from build123d import *

# Parameters (mm, degrees)
F0_R     = 10.5
F1_DEPTH = 14.2875
F3_DEPTH = 14.2875
F5_DEPTH = 14.2875


# Not quite as in the source:
# - a length typed as a fraction of an inch, garbled in the dataset ("3 / 203.2 mm" for 3/8 in), is restored
# - a feature names something its author has since deleted; it is built from what else it names


with BuildPart() as f1:
    # F0 (on Top) → F1 (new body)
    with BuildSketch(Plane.XY):
        with BuildLine():
            ThreePointArc((-84.5842045546, -55), (-80.1908062724, -65.6066017178), (-69.5842045546, -70))
            Line((-69.5842045546, -70), (69.5842045546, -70))
            ThreePointArc((69.5842045546, -70), (80.7788298305, -65.363034385), (85.4157954454, -54.1684091091))
            Line((85.4157954454, -54.1684091091), (85.4157954454, 66.6648875964))
            ThreePointArc((85.4157954454, 66.6648875964), (85.0717839963, 68.487460123), (84.0870871996, 70.0592383231))
            Line((84.0870871996, 70.0592383231), (-52.4659380977, 217.7534620916))
            ThreePointArc((-52.4659380977, 217.7534620916), (-55.9414029733, 219.3552750765), (-59.5315805785, 218.030403119))
            Line((-59.5315805785, 218.030403119), (-66.8741640868, 211.2417016656))
            Line((-66.8741640868, 211.2417016656), (-53.29676118, 196.556534649))
            Line((-53.29676118, 196.556534649), (-63.9435072671, 186.7129175415))
            Line((-63.9435072671, 186.7129175415), (-74.5902533541, 176.8693004341))
            Line((-74.5902533541, 176.8693004341), (-88.1676562609, 191.5544674507))
            Line((-88.1676562609, 191.5544674507), (-97.2821017235, 183.1275630663))
            ThreePointArc((-97.2821017235, 183.1275630663), (-98.5895263572, 181.1572441104), (-98.845348912, 178.8064844924))
            Line((-98.845348912, 178.8064844924), (-84.6266066394, 70.3235099279))
            ThreePointArc((-84.6266066394, 70.3235099279), (-84.5948163368, 69.9993075241), (-84.5842045546, 69.673723108))
            Line((-84.5842045546, 69.673723108), (-84.5842045546, -55))
        make_face()
        with Locations((-40, 0)):
            Circle(F0_R, mode=Mode.SUBTRACT)
        with Locations((40, 0)):
            Circle(F0_R, mode=Mode.SUBTRACT)
    extrude(amount=F1_DEPTH)

    # F2 (on face) → F3 (join)
    with BuildSketch(Plane(origin=(0, 0, 0), x_dir=(1, 0, 0), z_dir=(0, 0, -1))):
        with BuildLine():
            ThreePointArc((111.2211793661, 61.8855160475), (109.756713272, 65.4210499534), (106.2211793661, 66.8855160475))
            Line((106.2211793661, 66.8855160475), (79.0136510523, 66.8855160475))
            ThreePointArc((79.0136510523, 66.8855160475), (83.7249684911, 61.287261926), (85.4157954454, 54.1684091091))
            Line((85.4157954454, 54.1684091091), (85.4157954454, 37.1908284724))
            Line((85.4157954454, 37.1908284724), (111.2211793661, 37.1908284724))
            Line((111.2211793661, 37.1908284724), (111.2211793661, 61.8855160475))
        make_face()
        with BuildLine():
            ThreePointArc((85.4157954454, 54.1684091091), (83.7249684911, 61.287261926), (79.0136510523, 66.8855160475))
            Line((79.0136510523, 66.8855160475), (-78.7348607215, 66.8855160475))
            ThreePointArc((-78.7348607215, 66.8855160475), (-83.0426562208, 61.623449158), (-84.5842045546, 55))
            Line((-84.5842045546, 55), (-84.5842045546, 37.1908284724))
            Line((-84.5842045546, 37.1908284724), (85.4157954454, 37.1908284724))
            Line((85.4157954454, 37.1908284724), (85.4157954454, 54.1684091091))
        make_face()
        with BuildLine():
            ThreePointArc((-84.5842045546, 55), (-83.0426562208, 61.623449158), (-78.7348607215, 66.8855160475))
            Line((-78.7348607215, 66.8855160475), (-105.4471534491, 66.8855160475))
            ThreePointArc((-105.4471534491, 66.8855160475), (-108.982687355, 65.4210499534), (-110.4471534491, 61.8855160475))
            Line((-110.4471534491, 61.8855160475), (-110.4471534491, 37.1908284724))
            Line((-110.4471534491, 37.1908284724), (-84.5842045546, 37.1908284724))
            Line((-84.5842045546, 37.1908284724), (-84.5842045546, 55))
        make_face()
    extrude(amount=F3_DEPTH)

    # F4 (on face) → F5 (join)
    with BuildSketch(Plane(origin=(0, 0, 0), x_dir=(1, 0, 0), z_dir=(0, 0, -1))):
        with BuildLine():
            Line((111.2211793661, -36.8091715276), (-110.9449085174, -36.8091715276))
            Line((-110.9449085174, -36.8091715276), (-110.9449085174, -61.5038591027))
            ThreePointArc((-110.9449085174, -61.5038591027), (-109.4218951426, -65.0969864325), (-105.7806829141, -66.5011613701))
            Line((-105.7806829141, -66.5011613701), (-102.4463273268, -66.3915849369))
            ThreePointArc((-102.4463273268, -66.3915849369), (-98.8051150983, -67.7957598744), (-97.2821017235, -71.3888872042))
            Line((-97.2821017235, -71.3888872042), (-97.2821017235, -183.1275630663))
            Line((-97.2821017235, -183.1275630663), (-88.1676562609, -191.5544674507))
            Line((-88.1676562609, -191.5544674507), (-74.5902533541, -176.8693004341))
            Line((-74.5902533541, -176.8693004341), (-53.29676118, -196.556534649))
            Line((-53.29676118, -196.556534649), (-66.8741640868, -211.2417016656))
            Line((-66.8741640868, -211.2417016656), (-58.6359989162, -218.8584272777))
            Line((-58.6359989162, -218.8584272777), (58.8349498664, -91.8031638881))
            ThreePointArc((58.8349498664, -91.8031638881), (59.8196466631, -90.2313856879), (60.1636581123, -88.4088131614))
            Line((60.1636581123, -88.4088131614), (60.1636581123, -71.5038591027))
            ThreePointArc((60.1636581123, -71.5038591027), (61.6281242064, -67.9683251968), (65.1636581123, -66.5038591027))
            Line((65.1636581123, -66.5038591027), (106.2211793661, -66.5038591027))
            ThreePointArc((106.2211793661, -66.5038591027), (109.756713272, -65.0393930087), (111.2211793661, -61.5038591027))
            Line((111.2211793661, -61.5038591027), (111.2211793661, -36.8091715276))
        make_face()
    extrude(amount=F5_DEPTH)


solid = f1.part
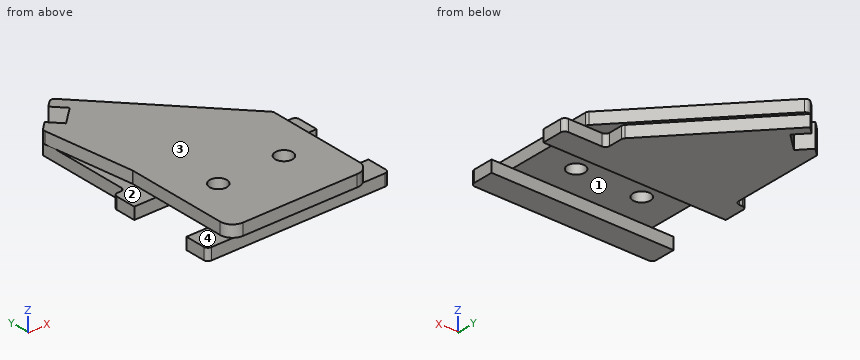
Can you work these out from the model? Positions are in its coordinate system, mm. Face numbers are marked on the shaded views. A direction names the side the tool comes from. Coordinates: 2 decimals unless noted, no trailing zeros. Order: outer loops, then holes, each group sorted by start corner. A loop starts at its lowest first (then second) coordinate and runs counter-clockwise, first axis right, second up. Notation, with made-up numbers: M -20,-13 L 22,-13 A22 cw 22,10 Z; hole C 73,-37 d10. An arc over 180 degrees is marked long. Write item = value, one per line.
(1) Suppose I cut it at C-C on x = -40. Please give me the cut outline in (y, z), plus the area to 3 significant figures.
Results are:
outline = M -70,0 L -66.89,0 L -66.89,-14.29 L -37.19,-14.29 L -37.19,0 L -10.5,0 L -10.5,14.29 L -70,14.29 Z; M 10.5,0 L 36.81,0 L 36.81,-14.29 L 198.7,-14.29 L 198.7,0 L 204.27,0 L 204.27,14.29 L 10.5,14.29 Z
area = 6,360 mm2
(2) I need wall thicknesses on line 1 along Y through (x, z) = (-66, -4.5); line 2 along Y through (x, z) = (59.5, -2); line 3 along Z through (x, y) = (51, -3). Which ranges of each line are inside material? Lowest first, please. Write a range as [from, to].
Results are:
line_1 = [-66.89, -37.19], [36.81, 184.81], [210.3, 212.05]
line_2 = [-66.89, -37.19], [36.81, 90.9]
line_3 = [0, 14.29]
(3) Suppose I cut it at D-D on y = 112. Please give me the cut outline in (x, z).
Results are:
outline = M -97.28,-14.29 L 40.16,-14.29 L 40.16,0 L 45.31,0 L 45.31,14.29 L -90.09,14.29 L -90.09,0 L -97.28,0 Z
(4) For pin 1 Ø11.5 at (y, z) = (128, -7.5) entering from -X; pin 2 Ø8 at (x, z) = (-3.5, -5.5) entering from +Y; pin 3 Ø1.3 at (x, y) = (-98, 175.5) entering from -Z; pin 4 Ø8 at (y, z) = (4.5, -7.5) entering from -X, each with a flat end and sliding along its axis, tell me the tip position at first contact or that it passes through.
Results are:
pin_1 = -97.28
pin_2 = 163.55
pin_3 = 0
pin_4 = through
(5) If we mould it in two halves opening along Y, with no side actions, what happens to the marked faces 1 and 2? For each: pulls with the +Y half, pulls with the -Y half, needs draft (parallel to the pull), parting line crosses it, or undercut.
Results are:
face_1 = undercut
face_2 = needs draft
(6) Suppose I cut it at B-B on y = 42. Please give me the cut outline in (x, z), plus the area to 3 significant figures.
Results are:
outline = M -110.94,-14.29 L 111.22,-14.29 L 111.22,0 L 85.42,0 L 85.42,14.29 L -84.58,14.29 L -84.58,0 L -110.94,0 Z
area = 5,600 mm2
(7) Suppose I cut it at A-A on z = -4.5. Please give me the cut outline in (x, y).
Results are:
outline = M -110.94,36.81 L 111.22,36.81 L 111.22,61.5 A5 ccw 106.22,66.5 L 65.16,66.5 A5 cw 60.16,71.5 L 60.16,88.41 A5 ccw 58.83,91.8 L -58.64,218.86 L -66.87,211.24 L -53.3,196.56 L -74.59,176.87 L -88.17,191.55 L -97.28,183.13 L -97.28,71.39 A5 cw -102.45,66.39 L -105.78,66.5 A5 ccw -110.94,61.5 Z; M -110.45,-61.89 A5 ccw -105.45,-66.89 L 106.22,-66.89 A5 ccw 111.22,-61.89 L 111.22,-37.19 L -110.45,-37.19 Z
(8) For the marked faces 3 and 4, which set-ups out of +Z, -Z, +X, -X, +Y, -Y let a thin tool reach every point of the face, with its end or its side?
Results are:
face_3 = +Z, +X, -X, +Y, -Y
face_4 = +Z, -X, -Y
